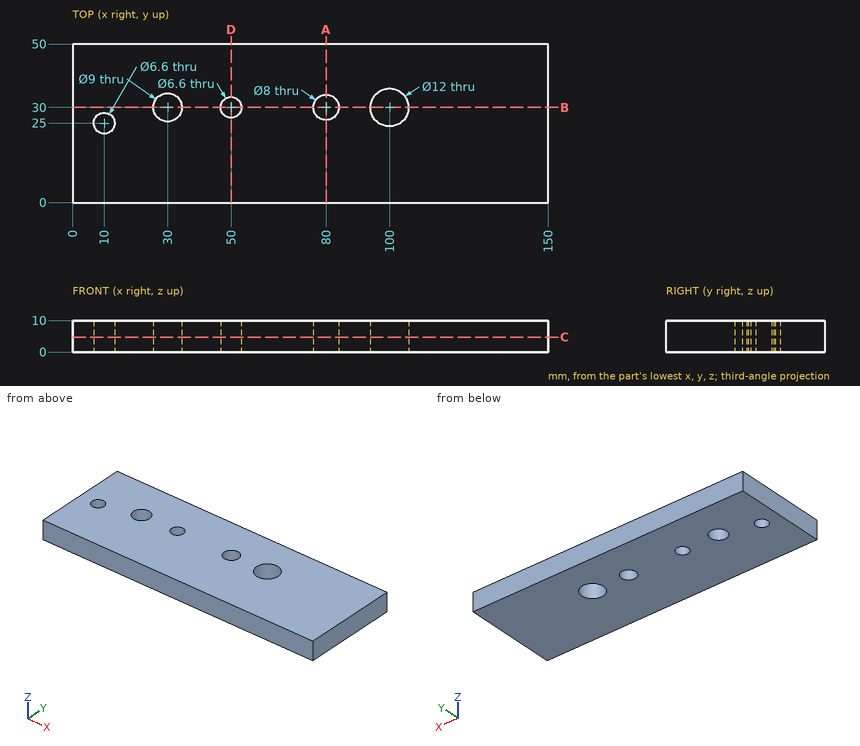
Design review of the part shown in the three views and the two pictorial views. Dimensions are in mm from the part's minimum x, y and z. Coordinates: 2 decimals unless noted, no trailing zeros. Order: outer loops, then holes, each group sorted by start corner. A loop starts at its lowest first (then second) coordinate and runs counter-clockwise, first axis right, second up. Notation, with made-up numbers: (-39, -22) - (16, -22) arc R19 cw to (16, 5) - close; hole circle Ø6 at (-22.5, -17.75). An arc over 180 degrees is marked (long way). One line per question, with ' | ' between items.
Q1. Consider section A-A, the plane x = 80. Give the boundary of the cut face in (y, z).
Answer key:
outline: (0, 0) - (26, 0) - (26, 10) - (0, 10) - close; (34, 0) - (50, 0) - (50, 10) - (34, 10) - close
Q2. Consider section B-B, the plane y = 30. Give the boundary of the cut face in (x, z).
Answer key:
outline: (0, 0) - (25.5, 0) - (25.5, 10) - (0, 10) - close; (34.5, 0) - (46.7, 0) - (46.7, 10) - (34.5, 10) - close; (53.3, 0) - (76, 0) - (76, 10) - (53.3, 10) - close; (84, 0) - (94, 0) - (94, 10) - (84, 10) - close; (106, 0) - (150, 0) - (150, 10) - (106, 10) - close
Q3. Consider section D-D, the plane x = 50. Give the boundary of the cut face in (y, z), then the cut area to 3 significant figures.
Answer key:
outline: (0, 0) - (26.7, 0) - (26.7, 10) - (0, 10) - close; (33.3, 0) - (50, 0) - (50, 10) - (33.3, 10) - close | area: 434 mm2
Q4. Consider section C-C, the plane z = 4.75. Give the boundary of the cut face in (x, y).
Answer key:
outline: (0, 0) - (150, 0) - (150, 50) - (0, 50) - close; hole circle Ø6.6 at (10, 25); hole circle Ø9 at (30, 30); hole circle Ø6.6 at (50, 30); hole circle Ø8 at (80, 30); hole circle Ø12 at (100, 30)
Q5. To check wall thickness, follow line 1 along X through (y, z) = (30, 2); line 2 along Y through (x, z) = (10, 2); line 3 along Y through (x, z) = (100, 5). State the ranges of each line that lie inside material, in increasing order.
Answer key:
line 1: x = 0 to 25.5, 34.5 to 46.7, 53.3 to 76, 84 to 94, 106 to 150 | line 2: y = 0 to 21.7, 28.3 to 50 | line 3: y = 0 to 24, 36 to 50
